```python
from build123d import *

# Parameters (mm, degrees)
F0_R     = 3.5
F1_DEPTH = 1
F2_DEPTH = 2


with BuildPart() as f1:
    # F0 (on Front) → F1 (new body)
    with BuildSketch(Plane.XZ):
        with BuildLine():
            Line((3.014297, 30.287076), (15.75, 31.5))
            Line((15.75, 31.5), (28.485703, 30.287076))
            ThreePointArc((28.485703, 30.287076), (29.710299, 29.710299), (30.287076, 28.485703))
            Line((30.287076, 28.485703), (31.454853, 16.224045))
            ThreePointArc((31.454853, 16.224045), (31.477375, 15.75), (31.454853, 15.275955))
            Line((31.454853, 15.275955), (30.287076, 3.014297))
            ThreePointArc((30.287076, 3.014297), (29.710299, 1.789701), (28.485703, 1.212924))
            Line((28.485703, 1.212924), (20.85, 0.485714))
            Line((20.85, 0.485714), (20.85, -1.523336))
            Line((20.85, -1.523336), (28.675321, -0.778067))
            ThreePointArc((28.675321, -0.778067), (31.124512, 0.375488), (32.278067, 2.824679))
            Line((32.278067, 2.824679), (33.445844, 15.086336))
            ThreePointArc((33.445844, 15.086336), (33.477375, 15.75), (33.445844, 16.413664))
            Line((33.445844, 16.413664), (32.278067, 28.675321))
            ThreePointArc((32.278067, 28.675321), (31.124512, 31.124512), (28.675321, 32.278067))
            Line((28.675321, 32.278067), (15.75, 33.50905))
            Line((15.75, 33.50905), (2.824679, 32.278067))
            ThreePointArc((2.824679, 32.278067), (0.375488, 31.124512), (-0.778067, 28.675321))
            Line((-0.778067, 28.675321), (-1.945844, 16.413664))
            ThreePointArc((-1.945844, 16.413664), (-1.977375, 15.75), (-1.945844, 15.086336))
            Line((-1.945844, 15.086336), (-0.778067, 2.824679))
            ThreePointArc((-0.778067, 2.824679), (0.375488, 0.375488), (2.824679, -0.778067))
            Line((2.824679, -0.778067), (10.65, -1.523336))
            Line((10.65, -1.523336), (10.65, 0.485714))
            Line((10.65, 0.485714), (3.014297, 1.212924))
            ThreePointArc((3.014297, 1.212924), (1.789701, 1.789701), (1.212924, 3.014297))
            Line((1.212924, 3.014297), (0.045147, 15.275955))
            ThreePointArc((0.045147, 15.275955), (0.022625, 15.75), (0.045147, 16.224045))
            Line((0.045147, 16.224045), (1.212924, 28.485703))
            ThreePointArc((1.212924, 28.485703), (1.789701, 29.710299), (3.014297, 30.287076))
        make_face()
        with BuildLine():
            Line((28.485703, 30.287076), (15.75, 31.5))
            Line((15.75, 31.5), (3.014297, 30.287076))
            ThreePointArc((3.014297, 30.287076), (1.789701, 29.710299), (1.212924, 28.485703))
            Line((1.212924, 28.485703), (0.045147, 16.224045))
            ThreePointArc((0.045147, 16.224045), (0.022625, 15.75), (0.045147, 15.275955))
            Line((0.045147, 15.275955), (1.212924, 3.014297))
            ThreePointArc((1.212924, 3.014297), (1.789701, 1.789701), (3.014297, 1.212924))
            Line((3.014297, 1.212924), (10.65, 0.485714))
            Line((10.65, 0.485714), (15.75, 0))
            Line((15.75, 0), (20.85, 0.485714))
            Line((20.85, 0.485714), (28.485703, 1.212924))
            ThreePointArc((28.485703, 1.212924), (29.710299, 1.789701), (30.287076, 3.014297))
            Line((30.287076, 3.014297), (31.454853, 15.275955))
            ThreePointArc((31.454853, 15.275955), (31.477375, 15.75), (31.454853, 16.224045))
            Line((31.454853, 16.224045), (30.287076, 28.485703))
            ThreePointArc((30.287076, 28.485703), (29.710299, 29.710299), (28.485703, 30.287076))
        make_face()
        with BuildLine():
            Line((5.439205, 23.914393), (5, 26.882069))
            ThreePointArc((5, 26.882069), (5.302961, 28.026619), (6.341624, 28.594914))
            Line((6.341624, 28.594914), (15.75, 29.49095))
            Line((15.75, 29.49095), (25.158376, 28.594914))
            ThreePointArc((25.158376, 28.594914), (26.197039, 28.026619), (26.5, 26.882069))
            Line((26.5, 26.882069), (26.060795, 23.914393))
            ThreePointArc((26.060795, 23.914393), (24.717088, 21.471599), (22.103894, 20.5))
            Line((22.103894, 20.5), (15.75, 20.5))
            Line((15.75, 20.5), (9.396106, 20.5))
            ThreePointArc((9.396106, 20.5), (6.782912, 21.471599), (5.439205, 23.914393))
        make_face(mode=Mode.SUBTRACT)
        with BuildLine():
            ThreePointArc((6.341624, 28.594914), (5.302961, 28.026619), (5, 26.882069))
            Line((5, 26.882069), (5.439205, 23.914393))
            ThreePointArc((5.439205, 23.914393), (6.782912, 21.471599), (9.396106, 20.5))
            Line((9.396106, 20.5), (15.75, 20.5))
            Line((15.75, 20.5), (22.103894, 20.5))
            ThreePointArc((22.103894, 20.5), (24.717088, 21.471599), (26.060795, 23.914393))
            Line((26.060795, 23.914393), (26.5, 26.882069))
            ThreePointArc((26.5, 26.882069), (26.197039, 28.026619), (25.158376, 28.594914))
            Line((25.158376, 28.594914), (15.75, 29.49095))
            Line((15.75, 29.49095), (6.341624, 28.594914))
        make_face()
        with Locations((15.75, 25.5)):
            Circle(F0_R, mode=Mode.SUBTRACT)
        Polygon((15.75, 0), (10.65, 0.485714), (10.65, -1.523336), (15.75, -2.00905), (20.85, -1.523336), (20.85, 0.485714), align=None)
    extrude(amount=F1_DEPTH)

    # F0 (on Front) → F2 (join)
    with BuildSketch(Plane.XZ):
        with BuildLine():
            ThreePointArc((6.341624, 28.594914), (5.302961, 28.026619), (5, 26.882069))
            Line((5, 26.882069), (5.439205, 23.914393))
            ThreePointArc((5.439205, 23.914393), (6.782912, 21.471599), (9.396106, 20.5))
            Line((9.396106, 20.5), (15.75, 20.5))
            Line((15.75, 20.5), (22.103894, 20.5))
            ThreePointArc((22.103894, 20.5), (24.717088, 21.471599), (26.060795, 23.914393))
            Line((26.060795, 23.914393), (26.5, 26.882069))
            ThreePointArc((26.5, 26.882069), (26.197039, 28.026619), (25.158376, 28.594914))
            Line((25.158376, 28.594914), (15.75, 29.49095))
            Line((15.75, 29.49095), (6.341624, 28.594914))
        make_face()
        with Locations((15.75, 25.5)):
            Circle(F0_R, mode=Mode.SUBTRACT)
        with BuildLine():
            Line((3.014297, 30.287076), (15.75, 31.5))
            Line((15.75, 31.5), (28.485703, 30.287076))
            ThreePointArc((28.485703, 30.287076), (29.710299, 29.710299), (30.287076, 28.485703))
            Line((30.287076, 28.485703), (31.454853, 16.224045))
            ThreePointArc((31.454853, 16.224045), (31.477375, 15.75), (31.454853, 15.275955))
            Line((31.454853, 15.275955), (30.287076, 3.014297))
            ThreePointArc((30.287076, 3.014297), (29.710299, 1.789701), (28.485703, 1.212924))
            Line((28.485703, 1.212924), (20.85, 0.485714))
            Line((20.85, 0.485714), (20.85, -1.523336))
            Line((20.85, -1.523336), (28.675321, -0.778067))
            ThreePointArc((28.675321, -0.778067), (31.124512, 0.375488), (32.278067, 2.824679))
            Line((32.278067, 2.824679), (33.445844, 15.086336))
            ThreePointArc((33.445844, 15.086336), (33.477375, 15.75), (33.445844, 16.413664))
            Line((33.445844, 16.413664), (32.278067, 28.675321))
            ThreePointArc((32.278067, 28.675321), (31.124512, 31.124512), (28.675321, 32.278067))
            Line((28.675321, 32.278067), (15.75, 33.50905))
            Line((15.75, 33.50905), (2.824679, 32.278067))
            ThreePointArc((2.824679, 32.278067), (0.375488, 31.124512), (-0.778067, 28.675321))
            Line((-0.778067, 28.675321), (-1.945844, 16.413664))
            ThreePointArc((-1.945844, 16.413664), (-1.977375, 15.75), (-1.945844, 15.086336))
            Line((-1.945844, 15.086336), (-0.778067, 2.824679))
            ThreePointArc((-0.778067, 2.824679), (0.375488, 0.375488), (2.824679, -0.778067))
            Line((2.824679, -0.778067), (10.65, -1.523336))
            Line((10.65, -1.523336), (10.65, 0.485714))
            Line((10.65, 0.485714), (3.014297, 1.212924))
            ThreePointArc((3.014297, 1.212924), (1.789701, 1.789701), (1.212924, 3.014297))
            Line((1.212924, 3.014297), (0.045147, 15.275955))
            ThreePointArc((0.045147, 15.275955), (0.022625, 15.75), (0.045147, 16.224045))
            Line((0.045147, 16.224045), (1.212924, 28.485703))
            ThreePointArc((1.212924, 28.485703), (1.789701, 29.710299), (3.014297, 30.287076))
        make_face()
    extrude(amount=F2_DEPTH)


solid = f1.part
```
CAD build for the part. Positions are in the model's coordinates, mm. A direction names the side the tool comes from. Round coordinates to 2 decimals unless told otherwise and drop trailing zeros. Write each loop counter-clockwise with the first axis right and the second up, starting at its lowest first coordinate (ties: lowest second). Pieces come first, ordered by that corner, then holes. Notation, with made-up numbers: (19.25, -12.75) - (29.25, -12.75) arc R35 ccw to (29.25, 19.25) - close; hole circle Ø8 at (31.25, -24.5). An arc over 180 degrees is marked (long way). Return JSON: item names as keys, results as strings. Group by question number.
Item 1: Flat gauge pin, fed straight in: pin 1 Ø1.1 at (x, y) = (15, -1.5) entering from -Z. Where does the tip first touch, or does it go through?
Item 2: Band-saw the part on C-C on z = 12.5. List the corners of the cut face in (x, y).
Item 3: Mould opens along Z. For faces 1 (the face through (16, 0, 16)), 2 (the face through (32.854, -0.986, 8.87)), 3 (the face through (24.721, -1.493, 0.854)) say: +Z half, -Z half, draft (parallel to the pull), parting line (faces both ways), or undercut.
Item 4: Band-saw the part on D-D on x = 20. List the corners of the cut face in (y, z).
Item 5: 3-axis set-ups, long thin cutter, end or side, ignore diameter. For faces 4 (the face through (10.65, -1.5, -0.5)), 5 (the face through (0.35, -0.99, 0.4)), 6 (the face through (29.7, -1.49, 29.72)): which of +Z, -Z, +X, -X, +Y, -Y reach the whole face in a straight line?
Item 6: Probe probe 1 along Z at (x, y) = (15.75, -1.1); probe 2 along Z at (x, y) = (21.5, -1.5); probe 3 along Z at (x, y) = (15.75, -0.8). List the from-to ranges inside material, lowest first.
Item 7: Band-saw the part on A-A on y = -0.4. List the corners of the cut face in (x, z).
Item 8: Band-saw the part on B-B on z = 25.5. List the corners of the cut face in (x, y), plus the area to 3 significant figures.
Resolved:
{
 "1": {"pin 1": "stops at z = -1.96"},
 "2": {"outline": "(-1.7, -2) - (0.31, -2) - (0.31, -1) - (31.19, -1) - (31.19, -2) - (33.2, -2) - (33.2, 0) - (-1.7, 0) - close"},
 "3": {"face 1": "draft", "face 2": "-Z half", "face 3": "undercut"},
 "4": {"outline": "(-2, 20.5) - (-1, 20.5) - (-1, -1.6) - (0, -1.6) - (0, 33.1) - (-2, 33.1) - (-2, 31.1) - (-1, 31.1) - (-1, 29.09) - (-2, 29.09) - close"},
 "5": {"face 4": "-Z, -Y", "face 5": "-Z, -X, +Y, -Y", "face 6": "-Y"},
 "6": {"probe 1": "z = 20.5 to 22, 29 to 29.49, 31.5 to 33.51", "probe 2": "z = -1.46 to 0.55, 20.5 to 28.94, 30.95 to 32.96", "probe 3": "z = -2.01 to 22, 29 to 33.51"},
 "7": {"outline": "(-1.95, 15.09) - (-0.78, 2.82) arc R4 ccw to (2.82, -0.78) - (15.75, -2.01) - (28.68, -0.78) arc R4 ccw to (32.28, 2.82) - (33.45, 15.09) arc R7 ccw to (33.45, 16.41) - (32.28, 28.68) arc R4 ccw to (28.68, 32.28) - (15.75, 33.51) - (2.82, 32.28) arc R4 ccw to (-0.78, 28.68) - (-1.95, 16.41) arc R7 ccw to start; hole circle Ø7 at (15.75, 25.5)"},
 "8": {"outline": "(-1.08, -2) - (0.93, -2) - (0.93, -1) - (5.2, -1) - (5.2, -2) - (12.25, -2) - (12.25, 0) - (-1.08, 0) - close; (19.25, -2) - (26.3, -2) - (26.3, -1) - (30.57, -1) - (30.57, -2) - (32.58, -2) - (32.58, 0) - (19.25, 0) - close", "area": "44.8 mm²"}
}
